Verification items for the finished model (mm, model axes). A direction names the side the tool comes from. Give positions to 0.01 mm unless a question says otherwise; leave off trailing zeros. Order: outer loops, then holes, each group sorted by start corner. A loop starts at its lowest first (then second) coordinate and runs counter-clockwise, first axis right, second up.
(1) Mould release check, pull along Y, two halves, no side actions. Record for faces 1 (the face through (3, 9.3, 15.875)), 2 (the face through (1.465, 24.171, 2.379)), 3 (the face through (14.274, -0.628, 11.046)): pulls with the +Y half, pulls with the -Y half, needs draft (parallel to the pull), parting line crosses it, or undercut.
(2) Scan lines: L1, parallel to Y at x = 0, z = 2.5 (1 decimal); L2, parallel to X at y = 0, z = 8.5 (1 decimal). Record each from-to range of solid material in increasing order.
(3) Access from +Z, -Z, +X, -X, +Y, -Y to the whole of each face (thin tool, end or side, straight path). Record for faces 4 (the face through (7.559, 5.796, 8.049)), 5 (the face through (17, -1, 6.35)).
(4) Sectioned sample at D-D on x = 10.5. Record the cut outline in (y, z) (3 decimals).
(5) Sectioned sample at B-B on x = 0. Count the separate pieces of the cut face and the enclosed holes in it, plus the area to 3 significant figures.
(6) Gauge pin test, flat ends, axial feed: pin 1 (1 mm diameter, centred on y = 5, z = 4, fed in from +X); pin 2 (4 mm diameter, centred on x = -26, y = 0.5, fed in from +Z); pin 3 (6 mm diameter, centred on x = -14.5, z = 9.5, fed in from +Y). Record the tip position at first contact, or that the pin passes through.
```python
from build123d import *

# Parameters (mm, degrees)
F2_R     = 3.175
F3_DEPTH = 15.876
F4_SIZE  = 1.524


with BuildPart() as f1:
    # F0 (on Front) → F1 (revolve)
    with BuildSketch(Plane.XZ):
        Polygon((-39.6875, 0), (-9.525, 0), (-9.525, 15.875), (-14.2875, 15.875), (-14.2875, 6.35), (-39.6875, 6.35), align=None)
    revolve(axis=Axis((0, 0, 22.6741275327), (0, 0, 1)))

    # F2 (on Top) → F3 (cut, through all)
    with BuildSketch(Plane.XY):
        with Locations((0, 26.9875)):
            Circle(F2_R)
    extrude(amount=F3_DEPTH, mode=Mode.SUBTRACT)

    # F4
    f4_edges = [f1.edges().sort_by_distance(p)[0] for p in [
        (-3.175, 26.9875, 6.35),
    ]]
    chamfer(f4_edges, length=F4_SIZE)


solid = f1.part
```
Ans:
1. face 1: needs draft
1. face 2: undercut
1. face 3: parting line crosses it
2. L1: y = -39.7 to -9.5, 9.5 to 23.8, 30.2 to 39.7
2. L2: x = -14.3 to -9.5, 9.5 to 14.3
3. face 4: +Z, -Z
3. face 5: +Z
4. outline: (-38.273, 0) - (38.273, 0) - (38.273, 6.35) - (9.689, 6.35) - (9.689, 15.875) - (-9.689, 15.875) - (-9.689, 6.35) - (-38.273, 6.35) - close
5. separate pieces: 3
5. enclosed holes: 0
5. area: 431 mm2
6. pin 1: stops at x = 39.43
6. pin 2: stops at z = 6.35
6. pin 3: stops at y = 8.48
